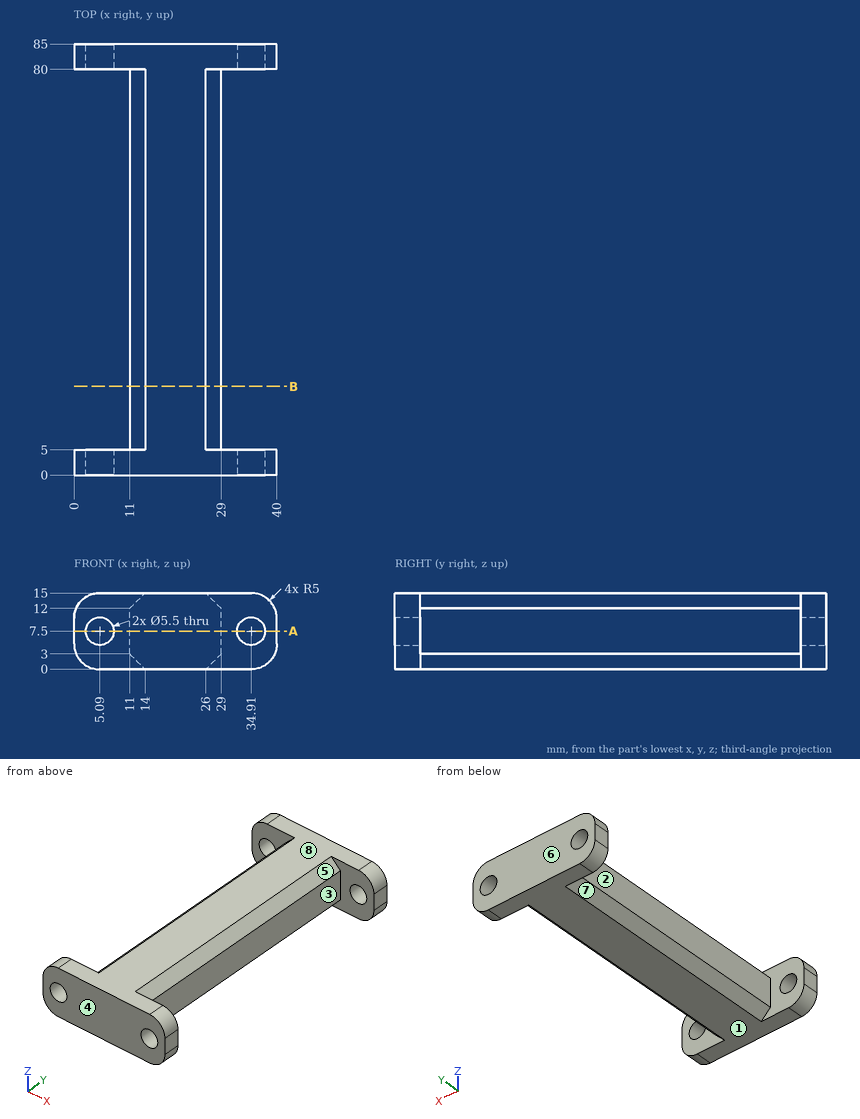
Print and shaded views of the part. All mm, measured from the part's lowest x, y and z. A direction names the side the tool comes from. Give positions to 0.01 mm unless a question says otherwise; leave off trailing zeros. Loops run counter-clockwise (first coordinate to the right, second up) from the corner with the lowest first, then second, coordinate; pieces in that order, holes last. Notation, with made-up numbers: (-7, 58.25) - (5, 58.25) arc R19 ccw to (5, 75.25) - close; hole circle Ø3 at (-6.5, -38.75). An arc over 180 degrees is marked (long way). One line per item, written item: value. Start each with the question number.
1. Which spindle directions (+Z, -Z, +X, -X, +Y, -Y) get a long thin tool onto all of the face, cutting with end or side? Do the marked faces 1, 2, 3, 4 and 5. Say none if no direction does.
2. Pull direction Y, two halves, no side cores. Call the marked faces 6, 7 and 8: pulls with the +Y half, pulls with the -Y half, needs draft (parallel to the pull), parting line crosses it, or undercut.
3. Slice it at A-A (z = 7.5). List the corners of the cut face in (x, y).
4. Pin check, flat tips, straight feed: pin 1 (6 mm diameter, centred on y = 18, z = 11.5, fed in from +X); pin 2 (2 mm diameter, centred on y = 70.5, z = 12.5, fed in from -X). Stop position of each tip, or through.
5. Slice it at B-B (y = 17.5). List the corners of the cut face in (x, z), plus the area to 3 significant figures.
6. Probe L1, parallel to Y at x = 8.5, z = 2.25; L2, parallel to Z at x = 34.91, y = 83.85; L3, parallel to X at y = 37, z = 4.25. List the from-to ranges inside material, lowest first. Write a range as from..to.
Solution:
1. face 1: -Z, +X, -X, +Y, -Y
1. face 2: +Z, -Z, -X
1. face 3: +Z, -Z, +X
1. face 4: +Z, -Z, +X, -X, -Y
1. face 5: +Z, +X
2. face 6: pulls with the +Y half
2. face 7: undercut
2. face 8: needs draft
3. outline: (0, 0) - (2.34, 0) - (2.34, 5) - (0, 5) - close; (0, 80) - (2.34, 80) - (2.34, 85) - (0, 85) - close; (7.84, 0) - (32.16, 0) - (32.16, 5) - (29, 5) - (29, 80) - (32.16, 80) - (32.16, 85) - (7.84, 85) - (7.84, 80) - (11, 80) - (11, 5) - (7.84, 5) - close; (37.66, 0) - (40, 0) - (40, 5) - (37.66, 5) - close; (37.66, 80) - (40, 80) - (40, 85) - (37.66, 85) - close
4. pin 1: stops at x = 29
4. pin 2: stops at x = 11
5. outline: (11, 3) - (14, 0) - (26, 0) - (29, 3) - (29, 12) - (26, 15) - (14, 15) - (11, 12) - close
5. area: 252 mm^2
6. L1: y = 0..5, 80..85
6. L2: z = 0..4.75, 10.25..15
6. L3: x = 11..29
